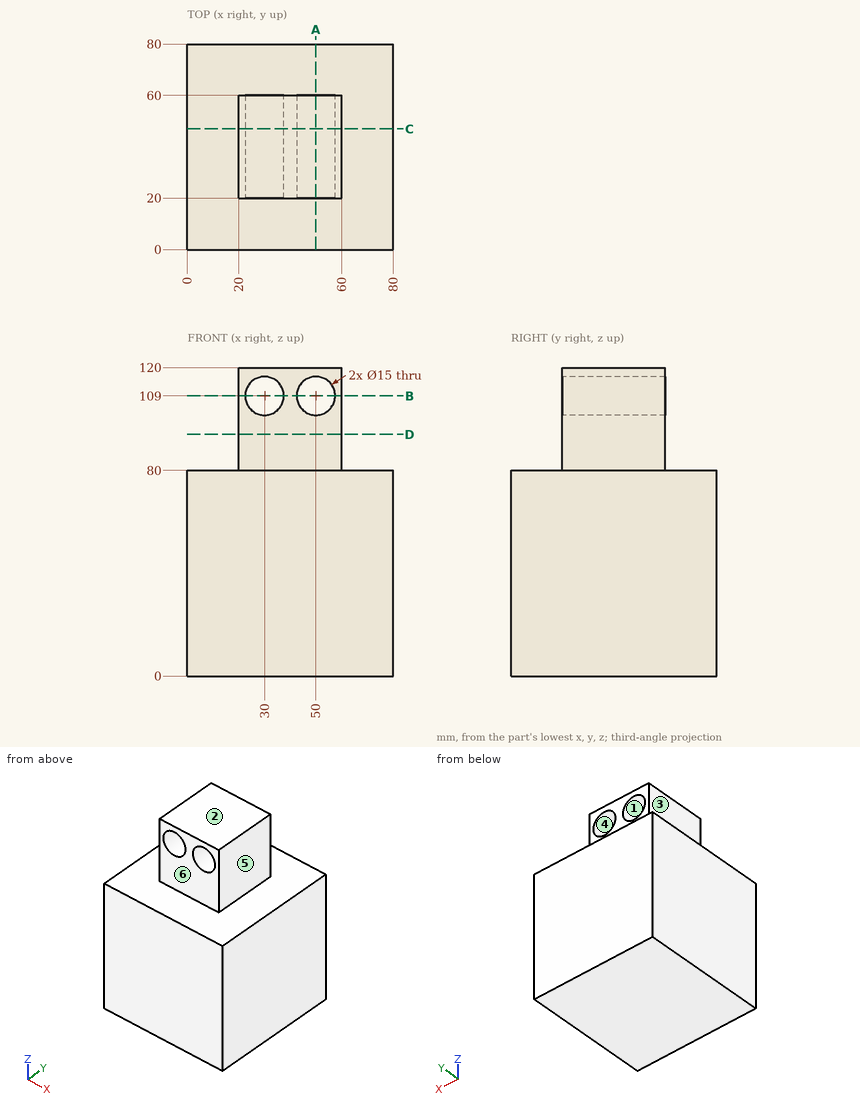
Design review of the part shown in the three views and the two pictorial views. Dimensions are in mm from the part's minimum x, y and z. A direction names the side the tool comes from. Round coordinates to 2 decimals unless told otherwise and drop trailing zeros. Loops run counter-clockwise (first coordinate to the right, second up) from the corner with the lowest first, then second, coordinate; pieces in that order, holes last.
(1) Tool access review of the marked faces 4, 5 and 6: name each direction out of +Z, -Z, +X, -X, +Y, -Y from which nothing blocks a thin tool from reaching the whole face with its end or side.
Returned:
face 4: +Y, -Y
face 5: +Z, +X, +Y, -Y
face 6: +Z, +X, -X, -Y
(2) Wall thickness on line 1 along X through (y, z) = (43, 104.5); line 2 along Z through (x, y) = (50, 30); line 3 along Z through (x, y) = (58, 10.5): over which ranges is each line inside the solid? List them lowest first.
Returned:
line 1: x = 20 to 24, 36 to 44, 56 to 60
line 2: z = 0 to 101.5, 116.5 to 120
line 3: z = 0 to 80
(3) We need section B-B (z = 109). Give the boundary of the cut face in (x, y).
Returned:
outline: (20, 20) - (22.5, 20) - (22.5, 60) - (20, 60) - close; (37.5, 20) - (42.5, 20) - (42.5, 60) - (37.5, 60) - close; (57.5, 20) - (60, 20) - (60, 60) - (57.5, 60) - close
(4) Mouldability with a two-part tool opening along Z and no side actions: class the marked faces 1, 2 and 3 as released by +Z, released by -Z, zero draft, split by the parting line, or undercut.
Returned:
face 1: undercut
face 2: released by +Z
face 3: zero draft
(5) We need section C-C (y = 47). Give the boundary of the cut face in (x, z), plus the area to 3 significant figures.
Returned:
outline: (0, 0) - (80, 0) - (80, 80) - (60, 80) - (60, 120) - (20, 120) - (20, 80) - (0, 80) - close; hole circle Ø15 at (30, 109); hole circle Ø15 at (50, 109)
area: 7,650 mm2
(6) We need section A-A (x = 50). Give the boundary of the cut face in (y, z), plus the area to 3 significant figures.
Returned:
outline: (0, 0) - (80, 0) - (80, 80) - (60, 80) - (60, 101.5) - (20, 101.5) - (20, 80) - (0, 80) - close; (20, 116.5) - (60, 116.5) - (60, 120) - (20, 120) - close
area: 7,400 mm2
(7) We need section D-D (z = 94). Give the boundary of the cut face in (x, y), plus the area to 3 significant figures.
Returned:
outline: (20, 20) - (60, 20) - (60, 60) - (20, 60) - close
area: 1,600 mm2
(8) Clearance check with flat-ended pins moving along their axes: P1, Ø1.5, axis at y = 32, z = 96, coming from the -X side; P2, Ø1.5, axis at x = 72, z = 13, coming from the -Y side; P3, Ø5, axis at x = 58.5, z = 106, coming from the +Y side; P4, Ø12, axis at x = 49.5, z = 95, coming from the -Y side. State where each tip first meets the part, or that it passes through.
Returned:
P1: stops at x = 20
P2: stops at y = 0
P3: stops at y = 60
P4: stops at y = 20
